from build123d import *

# Parameters (mm, degrees)
F0_W           = 150
F0_H           = 200
F0_W_2         = 137.5
F0_H_2         = 187.5
F0_R           = 5
F1_DEPTH       = 40
F3_DEPTH       = 155
F5_START       = -5
F5_DEPTH       = 140
F0_R_2         = 2.5
F6_DEPTH       = 5
F8_D           = 3
F8_CSINK_D     = 5
F8_CSINK_ANGLE = 90


with BuildPart() as f1:
    # F0 (on Top) → F1 (new body)
    with BuildSketch(Plane.XY):
        with Locations((2.626e-07, -0.2753496519)):
            Rectangle(F0_W, F0_H)
        with Locations((2.626e-07, -0.2753496519)):
            Rectangle(F0_W_2, F0_H_2, mode=Mode.SUBTRACT)
        with Locations((2.626e-07, -0.2753496519)):
            Rectangle(F0_W_2, F0_H_2)
        Polygon((-62.4999997374, 62.2246503481), (-62.4999997374, 87.2246503481), (-37.4999997374, 87.2246503481), (37.5000002626, 87.2246503481), (62.5000002626, 87.2246503481), (62.5000002626, 62.2246503481), (62.5000002626, -62.7753496519), (62.5000002626, -87.7753496519), (37.5000002626, -87.7753496519), (-37.4999997374, -87.7753496519), (-62.4999997374, -87.7753496519), (-62.4999997374, -62.7753496519), align=None, mode=Mode.SUBTRACT)
        Polygon((62.5000002626, 87.2246503481), (37.5000002626, 87.2246503481), (62.5000002626, 62.2246503481), align=None)
        with Locations((56.2500002626, 80.9746503481)):
            Circle(F0_R, mode=Mode.SUBTRACT)
        Polygon((-37.4999997374, 87.2246503481), (-62.4999997374, 87.2246503481), (-62.4999997374, 62.2246503481), align=None)
        with Locations((-56.2499997374, 80.9746503481)):
            Circle(F0_R, mode=Mode.SUBTRACT)
        Polygon((-37.4999997374, -87.7753496519), (-62.4999997374, -62.7753496519), (-62.4999997374, -87.7753496519), align=None)
        with Locations((-56.2499997374, -81.5253496519)):
            Circle(F0_R, mode=Mode.SUBTRACT)
        Polygon((62.5000002626, -87.7753496519), (62.5000002626, -62.7753496519), (37.5000002626, -87.7753496519), align=None)
        with Locations((56.2500002626, -81.5253496519)):
            Circle(F0_R, mode=Mode.SUBTRACT)
    extrude(amount=F1_DEPTH)

    # F2 (on face) → F3 (cut)
    with BuildSketch(Plane.YZ.offset(75.0000002626)):
        Polygon((99.7246503481, 40), (-100.2753496519, 40), (-100.2753496519, 10), align=None)
    extrude(amount=-F3_DEPTH, mode=Mode.SUBTRACT)

    # F4 (on face) → F5 (cut)
    with BuildSketch(Plane.YZ.offset(75.0000002626).offset(F5_START)):
        Polygon((94.7246503481, 39.25), (-95.2753496519, 10.75), (-95.2753496519, 5.75), (94.7246503481, 34.25), align=None)
    extrude(amount=-F5_DEPTH, mode=Mode.SUBTRACT)

    # F0 (on Top) → F6 (join)
    with BuildSketch(Plane.XY):
        with Locations((-56.2499997374, 80.9746503481)):
            Circle(F0_R)
        with Locations((-56.2499997374, 80.9746503481)):
            Circle(F0_R_2, mode=Mode.SUBTRACT)
        with Locations((56.2500002626, 80.9746503481)):
            Circle(F0_R)
        with Locations((56.2500002626, 80.9746503481)):
            Circle(F0_R_2, mode=Mode.SUBTRACT)
        with Locations((56.2500002626, -81.5253496519)):
            Circle(F0_R)
        with Locations((56.2500002626, -81.5253496519)):
            Circle(F0_R_2, mode=Mode.SUBTRACT)
        with Locations((-56.2499997374, -81.5253496519)):
            Circle(F0_R)
        with Locations((-56.2499997374, -81.5253496519)):
            Circle(F0_R_2, mode=Mode.SUBTRACT)
    extrude(amount=F6_DEPTH)

    # F8 (through all)
    with Locations(Plane(origin=(0, -2.9400443689, 19.6002957925), x_dir=(1, 0, 0), z_dir=(0, -0.1483404529, 0.9889363529))):
        with Locations((-62.4999997374, -85.7843935426), (-62.4999997374, 91.1734050987), (62.5000002626, 91.1734050987), (62.5000002626, -85.7843935426)):
            CounterSinkHole(F8_D / 2, F8_CSINK_D / 2, counter_sink_angle=F8_CSINK_ANGLE)


solid = f1.part
Design review of the part built by this model. Coordinates are the model's own, in mm. A direction names the side the tool comes from. Round coordinates to 2 decimals unless told otherwise and drop trailing zeros. Order: outer loops, then holes, each group sorted by start corner. A loop starts at its lowest first (then second) coordinate and runs counter-clockwise, first axis right, second up.
1) Consider section B-B (y = -4). State the section outline as (x, z) points, plus the area to 3 significant figures.
The answers:
outline: (-75, 0) - (-62.5, 0) - (-62.5, 19.44) - (-70, 19.44) - (-70, 24.44) - (-75, 24.44) - close; (62.5, 0) - (75, 0) - (75, 24.44) - (70, 24.44) - (70, 19.44) - (62.5, 19.44) - close
area: 536 mm2
2) Consider section D-D (z = 17.5). Count the separate pieces of the cut face and the enclosed holes in it, plus the area to 3 significant figures.
The answers:
separate pieces: 1
enclosed holes: 4
area: 5,270 mm2
3) Clearance check with flat-ended pins moving along their axes: pin 1 Ø16 at (x, y) = (-56.25, -81.53) entering from +Z; pin 2 Ø8 at (x, y) = (56.25, 80.97) entering from +Z; pin 3 Ø1.5 at (x, z) = (-14.5, 25) entering from -Y; pin 4 Ø8 at (x, y) = (-56.25, 80.97) entering from -Z. State where each tip first meets the part, or that it passes through.
The answers:
pin 1: stops at z = 9.01
pin 2: stops at z = 5
pin 3: stops at y = 87.22
pin 4: stops at z = 0
4) Machinability: for faces 1 (the flat face through (-49.825, -75.45, 4.058)), 2 (the cylindrical face through (61.694, 91.088, 15.895)), 3 (the cylindrical face through (-53.56, 85.19, 18.81)), which of the approach directions +Z, -Z, +X, -X, +Y, -Y give a long, thin tool a straight path to every point of the face, cutting with its end or side? Answer none if there is none.
The answers:
face 1: +Z, -Z
face 2: none
face 3: +Z
5) Consider section C-C (x = -56.25). State the section outline as (y, z) points.
The answers:
outline: (-100.28, 0) - (-84.03, 0) - (-84.03, 5) - (-86.53, 5) - (-86.53, 7.06) - (-95.28, 5.75) - (-95.28, 10.75) - (-100.28, 10) - close; (-79.03, 0) - (-69.03, 0) - (-69.03, 9.69) - (-76.53, 8.56) - (-76.53, 5) - (-79.03, 5) - close; (68.47, 0) - (78.47, 0) - (78.47, 5) - (75.97, 5) - (75.97, 31.44) - (68.47, 30.31) - close; (83.47, 0) - (99.72, 0) - (99.72, 40) - (94.72, 39.25) - (94.72, 34.25) - (85.97, 32.94) - (85.97, 5) - (83.47, 5) - close
6) For L1, parallel to X at y = 43, z = 31; L2, parallel to X at y = 50, z = 13.5; L3, parallel to Y at x = -26, z = 4, list the stretches that pass through material, from the lowest coordinate up.
The answers:
L1: x = -75 to -70, 70 to 75
L2: x = -75 to -62.5, 62.5 to 75
L3: y = -100.28 to -87.78, 87.22 to 99.72
7) Consider section A-A (x = -23.5). State the section outline as (y, z) points (3 decimals).
The answers:
outline: (-100.275, 0) - (-87.775, 0) - (-87.775, 6.875) - (-95.275, 5.75) - (-95.275, 10.75) - (-100.275, 10) - close; (87.225, 0) - (99.725, 0) - (99.725, 40) - (94.725, 39.25) - (94.725, 34.25) - (87.225, 33.125) - close
